For this review, take the finished solid that the model builds, in its own axes (mm). A direction names the side the tool comes from. Coordinates: 2 decimals unless noted, no trailing zeros. Loops run counter-clockwise (first coordinate to the right, second up) from the corner with the lowest first, then second, coordinate; pieces in that order, holes last. Notation, with made-up numbers: (-1.5, 42.5) -> (23.5, 42.5) arc R19 ccw to (23.5, 66.5) -> close; hole circle Ø11 at (50.5, -23). An arc over 180 degrees is marked (long way). One line per item, written item: value.
from build123d import *

# Parameters (mm, degrees)
F0_W     = 76
F0_H     = 6
F1_DEPTH = 7
F2_W     = 76.920286
F2_H     = 6
F3_DEPTH = 2.237
F5_DEPTH = 76.001
F6_SIZE  = 0.1
F7_W     = 58.94864
F7_H     = 6
F8_DEPTH = 1


with BuildPart() as f1:
    # F0 (on Top) → F1 (new body)
    with BuildSketch(Plane.XY):
        Rectangle(F0_W, F0_H)
    extrude(amount=F1_DEPTH)

    # F2 (on face) → F3 (cut)
    with BuildSketch(Plane.XY.offset(7)):
        with Locations((0.460143, 0)):
            Rectangle(F2_W, F2_H)
    extrude(amount=-F3_DEPTH, mode=Mode.SUBTRACT)

    # F4 (on face) → F5 (cut, through all)
    with BuildSketch(Plane.YZ.offset(38)):
        with BuildLine():
            Line((1.437258, 7), (-1.437258, 7))
            Line((-1.437258, 7), (-0.109352, 4.7))
            Line((-0.109352, 4.7), (-0.046194, 4.547522))
            ThreePointArc((-0.046194, 4.547522), (0, 4.516656), (0.046194, 4.547522))
            Line((0.046194, 4.547522), (0.109352, 4.7))
            Line((0.109352, 4.7), (1.437258, 7))
        make_face()
    extrude(amount=-F5_DEPTH, mode=Mode.SUBTRACT)

    # F6
    f6_edges = [f1.edges().sort_by_distance(p)[0] for p in [
        (0, -3, 0),
        (38, 0, 0),
        (0, 3, 0),
        (-38, 0, 0),
        (-38, -1.572863, 4.763),
        (-38, 1.572863, 4.763),
    ]]
    chamfer(f6_edges, length=F6_SIZE)

    # F7 (on face) → F8 (cut)
    with BuildSketch(Plane.XY.offset(4.763)):
        with Locations((-11.47432, 0)):
            Rectangle(F7_W, F7_H)
    extrude(amount=-F8_DEPTH, mode=Mode.SUBTRACT)


solid = f1.part
1. To check wall thickness, follow probe 1 along Z at (x, y) = (-10, -1.3); probe 2 along X at (y, z) = (0.8, 4.4); probe 3 along Z at (x, y) = (19, 0). State the ranges of each line that lie inside material, in increasing order. Write a range as from..to.
Return value:
probe 1: z = 0..3.76
probe 2: x = 18..38
probe 3: z = 0..4.52
2. Take a section at B-B, the plane x = -6. Give the boundary of the cut face in (y, z), and give its area (3 significant figures).
Return value:
outline: (-3, 0.1) -> (-2.9, 0) -> (2.9, 0) -> (3, 0.1) -> (3, 3.76) -> (-3, 3.76) -> close
area: 22.6 mm2
3. For faces 1 (the flat face through (38, 0, 2)), 2 (the flat face through (-10, 0, 3.763)), list the 3-axis set-ups (+Z, -Z, +X, -X, +Y, -Y) from which the entire face can be reached by the end or side of a thin tool; tool diameter is ignored.
Return value:
face 1: +Z, -Z, +X, +Y, -Y
face 2: +Z, -X, +Y, -Y
4. Insertion check: pin 1 Ø3 at (x, y) = (12, 1.5) entering from +Z; pin 2 Ø1.1 at (y, z) = (-1.5, 4.5) entering from -X. Each pin has a flat end and moves straight along its axis. Give the tip position at first contact, or say it passes through.
Return value:
pin 1: stops at z = 3.76
pin 2: stops at x = 18
5. Take a section at A-A, the plane y = 2.15. Give the boundary of the cut face in (x, z), and give its area (3 significant figures).
Return value:
outline: (-38, 0.1) -> (-37.9, 0) -> (37.9, 0) -> (38, 0.1) -> (38, 4.76) -> (18, 4.76) -> (18, 3.76) -> (-38, 3.76) -> close
area: 306 mm2
